Build history of the part. All positions in model axes, mm. A direction names the side the tool comes from. Round coordinates to 2 decimals unless told otherwise and drop trailing zeros. Write each loop counter-clockwise with the first axis right and the second up, starting at its lowest first coordinate (ties: lowest second). Pieces come first, ordered by that corner, then holes.
Item 1: 3-axis set-ups, long thin cutter, end or side, ignore diameter. For faces 1 (the cylindrical face through (40.3, -36.1, 4.5)), 2 (the flat face through (-31, 11, 6)), 3 (the flat face through (28, 27, 4)): which of +Z, -Z, +X, -X, +Y, -Y reach the whole face in a straight line?
Item 2: Band-saw the part on B-B, the plane x = 40.25. Write the cut outline in (y, z), then the cut area to 3 significant figures.
Item 3: Band-saw the part on A-A, the plane y = 36. Count the separate pieces of the cut face and the enclosed holes in it, then the cut area to 3 significant figures.
Item 4: Drop flat-ended pins along their axis: pin 1 Ø0.8 at (y, z) = (47, 5) entering from -X; pin 2 Ø0.8 at (x, y) = (1, 47) entering from +Z; pin 3 Ø1.8 at (x, z) = (-33, 4) entering from +Y. Give the stop position or say it passes through.
Item 5: Mould opens along Y. For faces 4 (the flat face through (-3, 32.5, 6)), 5 (the flat face through (40, -42.5, 4)), 6 (the flat face through (-34, 38, 4)), 7 (the flat face through (-29, 10, 6)) say: +Y half, -Y half, draft (parallel to the pull), parting line (faces both ways), or undercut.
Item 6: Band-saw the part on C-C, the plane x = 21. Write the cut outline in (y, z), then the cut area to 3 significant figures.
Item 7: Band-saw the part on D-D, the plane y = -38.5. Write the cut outline in (x, z).
Item 8: Wall check: probe 1 along X at (y, z) = (37, 2.5); probe 2 along X at (y, z) = (11, 4.75); probe 3 along X at (y, z) = (41.5, 0.5). Give the ranges that are in metal, low to high.
```python
from build123d import *
from OCP.BRepAlgoAPI import BRepAlgoAPI_Cut
from OCP.TopTools import TopTools_ListOfShape

# Parameters (mm, degrees)
BOSS_EXTRUDE1_DEPTH = 7.5
CUT_EXTRUDE1_DEPTH  = 3.2
CUT_EXTRUDE2_DEPTH  = 5
CUT_EXTRUDE3_DEPTH  = 50
CUT_EXTRUDE4_REACH  = 70.655
SKETCH5_W           = 3
SKETCH5_H           = 17
CUT_EXTRUDE5_REACH  = 70.655
SKETCH8_W           = 12
SKETCH8_H           = 37
CUT_EXTRUDE6_DEPTH  = 3.2
SKETCH10_W          = 10
SKETCH10_H          = 7.5
BOSS_EXTRUDE2_DEPTH = 27.486353186
SKETCH11_W          = 3
SKETCH11_H          = 7.5
CUT_EXTRUDE7_DEPTH  = 3.5
SKETCH12_W          = 2
SKETCH12_H          = 7.5
CUT_EXTRUDE8_DEPTH  = 4
SKETCH13_W          = 2
SKETCH13_H          = 7.5
CUT_EXTRUDE9_DEPTH  = 4
SKETCH14_W          = 7.5
SKETCH14_H          = 9.5
CUT_EXTRUDE10_DEPTH = 6
SKETCH15_W          = 1.5
SKETCH15_H          = 21
SKETCH15_H_2        = 1
CUT_EXTRUDE11_DEPTH = 1.5
SKETCH16_W          = 1.5
SKETCH16_H          = 7.5
CUT_EXTRUDE12_DEPTH = 35.486360958


with BuildPart() as part:
    # Sketch1 → Boss-Extrude1 (new body)
    with BuildSketch(Plane.XY):
        with BuildLine():
            Line((-33, -47.5), (49, -47.5))
            Line((49, -47.5), (49, -29.5))
            Line((49, -29.5), (31.5, -29.5))
            Line((31.5, -29.5), (31.5, 2.5))
            Line((31.5, 2.5), (49, 2.5))
            Line((49, 2.5), (49, 47.5))
            Line((49, 47.5), (30, 47.5))
            Line((30, 47.5), (30, 30.5))
            Line((30, 30.5), (27, 30.5))
            Line((27, 30.5), (27, 47.5))
            Line((27, 47.5), (-49, 47.5))
            Line((-49, 47.5), (-49, -31.5))
            ThreePointArc((-49, -31.5), (-44.313708499, -42.813708499), (-33, -47.5))
        make_face()
    extrude(amount=BOSS_EXTRUDE1_DEPTH)

    # Sketch2 → Cut-Extrude1 (cut)
    with BuildSketch(Plane.XY.offset(7.5)):
        Polygon((30, 40), (31, 40), (31, 32.5), (36, 32.5), (36, 28.5), (38, 28.5), (38, 32.5), (48, 32.5), (48, 46.5), (38, 46.5), (38, 47.5), (36, 47.5), (36, 46.5), (31, 46.5), (31, 45), (30, 45), align=None)
        Polygon((-16, 40), (-15, 40), (-15, 32.5), (-10, 32.5), (-10, 28.5), (-8, 28.5), (-8, 32.5), (2, 32.5), (2, 46.5), (-8, 46.5), (-8, 47.5), (-10, 47.5), (-10, 46.5), (-15, 46.5), (-15, 45), (-16, 45), align=None)
        Polygon((7, 40), (8, 40), (8, 32.5), (13, 32.5), (13, 28.5), (15, 28.5), (15, 32.5), (25, 32.5), (25, 46.5), (15, 46.5), (15, 47.5), (13, 47.5), (13, 46.5), (8, 46.5), (8, 45), (7, 45), align=None)
    extrude(amount=-CUT_EXTRUDE1_DEPTH, mode=Mode.SUBTRACT)

    # Sketch3 → Cut-Extrude2 (cut)
    with BuildSketch(Plane.XZ.offset(47.5)):
        with BuildLine():
            Line((34.25, 7.5), (46.25, 7.5))
            ThreePointArc((46.25, 7.5), (40.25, 1.5), (34.25, 7.5))
        make_face()
    extrude(amount=-CUT_EXTRUDE2_DEPTH, mode=Mode.SUBTRACT)

    # Sketch4 → Cut-Extrude3 (cut)
    with BuildSketch(Plane.XZ.offset(42.5)):
        with BuildLine():
            Line((37.25, 7.5), (43.25, 7.5))
            ThreePointArc((43.25, 7.5), (40.25, 4.5), (37.25, 7.5))
        make_face()
    extrude(amount=-CUT_EXTRUDE3_DEPTH, mode=Mode.SUBTRACT)

    # Sketch5 → Cut-Extrude4 (cut, up to next)
    with BuildSketch(Plane.XY.offset(7.5), mode=Mode.PRIVATE) as cut_extrude4_sk1:
        with Locations((5.5, 39)):
            Rectangle(SKETCH5_W, SKETCH5_H)
    cut_extrude4_tool1 = extrude(cut_extrude4_sk1.sketch, amount=-CUT_EXTRUDE4_REACH, mode=Mode.PRIVATE) & part.part
    # Sketch5 → Cut-Extrude4 (cut, up to next)
    with BuildSketch(Plane.XY.offset(7.5), mode=Mode.PRIVATE) as cut_extrude4_sk2:
        with Locations((-17.5, 39)):
            Rectangle(SKETCH5_W, SKETCH5_H)
    cut_extrude4_tool2 = extrude(cut_extrude4_sk2.sketch, amount=-CUT_EXTRUDE4_REACH, mode=Mode.PRIVATE) & part.part
    add(cut_extrude4_tool1.solids().sort_by_distance((5.5, 39, 7.5))[0], mode=Mode.SUBTRACT)
    add(cut_extrude4_tool2.solids().sort_by_distance((-17.5, 39, 7.5))[0], mode=Mode.SUBTRACT)

    # Sketch8 → Cut-Extrude5 (cut, up to next)
    with BuildSketch(Plane.XY.offset(7.5), mode=Mode.PRIVATE) as cut_extrude5_sk1:
        with Locations((-43, 29)):
            Rectangle(SKETCH8_W, SKETCH8_H)
    cut_extrude5_tool1 = extrude(cut_extrude5_sk1.sketch, amount=-CUT_EXTRUDE5_REACH, mode=Mode.PRIVATE) & part.part
    add(cut_extrude5_tool1.solids().sort_by_distance((-43, 29, 7.5))[0], mode=Mode.SUBTRACT)

    # Sketch9 → Cut-Extrude6 (cut)
    with BuildSketch(Plane.XY.offset(7.5)):
        Polygon((-37, 20), (-36, 20), (-36, 12.5), (-31, 12.5), (-31, 8.5), (-29, 8.5), (-29, 12.5), (-19, 12.5), (-19, 26.5), (-29, 26.5), (-29, 30.5), (-31, 30.5), (-31, 26.5), (-36, 26.5), (-36, 25), (-37, 25), align=None)
    extrude(amount=-CUT_EXTRUDE6_DEPTH, mode=Mode.SUBTRACT)

    # Sketch10 → Boss-Extrude2 (add)
    with BuildSketch(Plane(origin=(0, 10.5, 0), x_dir=(1, 0, 0), z_dir=(0, 1, 0))):
        with Locations((-44, -3.75)):
            Rectangle(SKETCH10_W, SKETCH10_H)
    extrude(amount=BOSS_EXTRUDE2_DEPTH)

    # Sketch11 → Cut-Extrude7 (cut)
    with BuildSketch(Plane(origin=(0, 30.5, 0), x_dir=(1, 0, 0), z_dir=(0, 1, 0))):
        with Locations((-17.5, -3.75)):
            Rectangle(SKETCH11_W, SKETCH11_H)
        with Locations((5.5, -3.75)):
            Rectangle(SKETCH11_W, SKETCH11_H)
        with Locations((28.5, -3.75)):
            Rectangle(SKETCH11_W, SKETCH11_H)
    extrude(amount=-CUT_EXTRUDE7_DEPTH, mode=Mode.SUBTRACT)

    # Sketch12 → Cut-Extrude8 (cut)
    with BuildSketch(Plane(origin=(0, 10.5, 0), x_dir=(1, 0, 0), z_dir=(0, 1, 0))):
        with Locations((-38, -3.75)):
            Rectangle(SKETCH12_W, SKETCH12_H)
    extrude(amount=-CUT_EXTRUDE8_DEPTH, mode=Mode.SUBTRACT)

    # Sketch13 → Cut-Extrude9 (cut)
    with BuildSketch(Plane(origin=(0, 6.5, 0), x_dir=(1, 0, 0), z_dir=(0, 1, 0))):
        with Locations((-38, -3.75)):
            Rectangle(SKETCH13_W, SKETCH13_H)
    extrude(amount=-CUT_EXTRUDE9_DEPTH, mode=Mode.SUBTRACT)

    # Sketch14 → Cut-Extrude10 (cut)
    with BuildSketch(Plane.ZY.offset(37)):
        with Locations((3.75, 42.75)):
            Rectangle(SKETCH14_W, SKETCH14_H)
    extrude(amount=-CUT_EXTRUDE10_DEPTH, mode=Mode.SUBTRACT)

    # Sketch15 → Cut-Extrude11 (cut)
    with BuildSketch(Plane.XY.offset(7.5)):
        with Locations((-19.75, 37)):
            Rectangle(SKETCH15_W, SKETCH15_H)
        with Locations((1.25, 47)):
            Rectangle(SKETCH15_W, SKETCH15_H_2)
        with Locations((24.25, 47)):
            Rectangle(SKETCH15_W, SKETCH15_H_2)
        with Locations((47.25, 47)):
            Rectangle(SKETCH15_W, SKETCH15_H_2)
    extrude(amount=-CUT_EXTRUDE11_DEPTH, mode=Mode.SUBTRACT)


with BuildPart() as cut_extrude12_tool:
    # Sketch16 → Cut-Extrude12 (new body)
    with BuildSketch(Plane(origin=(0, 37.986353186, 0), x_dir=(1, 0, 0), z_dir=(0, 1, 0))):
        with Locations((-39.75, -3.75)):
            Rectangle(SKETCH16_W, SKETCH16_H)
    extrude(amount=-CUT_EXTRUDE12_DEPTH)


with BuildPart() as part_1:
    add(part.part)

    # Cut-Extrude12: cut by cut_extrude12_tool, with a tolerance
    cut_extrude12_stock = TopTools_ListOfShape()
    cut_extrude12_stock.Append(part_1.part.wrapped)
    cut_extrude12_tools = TopTools_ListOfShape()
    cut_extrude12_tools.Append(cut_extrude12_tool.part.wrapped)
    cut_extrude12_cut = BRepAlgoAPI_Cut()
    cut_extrude12_cut.SetArguments(cut_extrude12_stock)
    cut_extrude12_cut.SetTools(cut_extrude12_tools)
    cut_extrude12_cut.SetFuzzyValue(0.00001)
    cut_extrude12_cut.Build()
    add(Compound.cast(cut_extrude12_cut.Shape()).solids(), mode=Mode.REPLACE)


solid = part_1.part
```
Results:
1. face 1: +Z, -Y
1. face 2: +Z
1. face 3: +Z, -Z, +Y
2. outline: (-47.5, 0) - (-29.5, 0) - (-29.5, 4.5) - (-42.5, 4.5) - (-42.5, 1.5) - (-47.5, 1.5) - close; (2.5, 0) - (47.5, 0) - (47.5, 7.5) - (46.5, 7.5) - (46.5, 4.3) - (32.5, 4.3) - (32.5, 7.5) - (7.5, 7.5) - (7.5, 4.5) - (2.5, 4.5) - close
2. area: 344 mm2
3. separate pieces: 5
3. enclosed holes: 0
3. area: 476 mm2
4. pin 1: stops at x = -31
4. pin 2: stops at z = 6
4. pin 3: stops at y = 38
5. face 4: undercut
5. face 5: -Y half
5. face 6: +Y half
5. face 7: undercut
6. outline: (-47.5, 0) - (47.5, 0) - (47.5, 7.5) - (46.5, 7.5) - (46.5, 4.3) - (32.5, 4.3) - (32.5, 7.5) - (-47.5, 7.5) - close
6. area: 668 mm2
7. outline: (-47.39, 0) - (49, 0) - (49, 7.5) - (43.25, 7.5) arc R3 cw to (37.25, 7.5) - (-47.39, 7.5) - close
8. probe 1: x = -49 to -40.5, -37 to -19, -16 to 4, 7 to 27, 30 to 49
8. probe 2: x = -49 to -40.5, -37 to -31, -29 to 49
8. probe 3: x = -31 to -19, -16 to 4, 7 to 27, 30 to 49
